Can you work these out from the model? Positions are in its coordinate system, mm. A direction names the side the tool comes from. Give positions to 0.01 mm unless a question says otherwise; leave off trailing zeros. Write each loop counter-clockwise with the first axis right and the second up, starting at its lowest first coordinate (ties: lowest second). Pieces come first, ordered by that corner, then holes. Notation, with made-up numbers: (20.5, -11.5) - (73.5, -11.5) arc R18 ccw to (73.5, -5.5) - close; hole circle Ø10 at (-23.5, -3.75). An arc over 180 degrees is marked (long way). Return JSON: item names as keys, results as strings. Group by question number.
from build123d import *

# Parameters (mm, degrees)
F1_R     = 7.5
F1_W     = 13
F1_H     = 13
F2_DEPTH = 5


with BuildPart() as f2:
    # F1 (on Right) → F2 (new body)
    with BuildSketch(Plane.YZ):
        Polygon((0, 15), (0, 0), (30, 0), (30, -5), (35, -5), (35, 0), (43.5, 0), (43.5, 2), (42.25, 2), (42.25, 5), (43.5, 5), (43.5, 6), (46.5, 6), (46.5, 5), (47.75, 5), (47.75, 2), (46.5, 2), (46.5, 0), (55, 0), (55, -5), (60, -5), (60, 0), (90, 0), (90, 15), (95, 15), (95, 20), (90, 20), (90, 28.5), (88, 28.5), (88, 27.25), (85, 27.25), (85, 28.5), (84, 28.5), (84, 31.5), (85, 31.5), (85, 32.75), (88, 32.75), (88, 31.5), (90, 31.5), (90, 40), (95, 40), (95, 45), (90, 45), (90, 60), (60, 60), (60, 65), (55, 65), (55, 60), (46.5, 60), (46.5, 58), (47.75, 58), (47.75, 55), (46.5, 55), (46.5, 54), (43.5, 54), (43.5, 55), (42.25, 55), (42.25, 58), (43.5, 58), (43.5, 60), (35, 60), (35, 65), (30, 65), (30, 60), (0, 60), (0, 45), (-5, 45), (-5, 40), (0, 40), (0, 31.5), (2, 31.5), (2, 32.75), (5, 32.75), (5, 31.5), (6, 31.5), (6, 28.5), (5, 28.5), (5, 27.25), (2, 27.25), (2, 28.5), (0, 28.5), (0, 20), (-5, 20), (-5, 15), align=None)
        with Locations((20, 22)):
            Circle(F1_R, mode=Mode.SUBTRACT)
        with Locations((55.75, 13)):
            Rectangle(F1_W, F1_H, mode=Mode.SUBTRACT)
        with BuildLine():
            Line((25, 50), (65, 50))
            ThreePointArc((65, 50), (70, 45), (65, 40))
            Line((65, 40), (25, 40))
            ThreePointArc((25, 40), (20, 45), (25, 50))
        make_face(mode=Mode.SUBTRACT)
    extrude(amount=F2_DEPTH)


solid = f2.part
1) Imagine slicing it at B-B, the plane y = 66. Write out the boundary of the cut face in (x, z), and give its area (3 significant figures).
2) Will these pins go through, and if not, where does the flat tip stop? pin 1 Ø2.5 at (x, y) = (3.5, 42.5) entering from +Z; pin 2 Ø1.5 at (x, y) = (2, 3) entering from -Z; pin 3 Ø2.5 at (x, z) = (3, 56) entering from -Y; pin 4 Ø5 at (y, z) = (17.5, 52) entering from -X.
3) On a 3-axis mill with a long thin cutter (end or side, diameter ignored), from which of +Z, -Z, +X, -X, +Y, -Y can I reach the whole of each face in a straight line? I mean faces 1 (the face through (2, 56, 19.5)), 2 (the face through (2, -2, 20)), 3 (the face through (2, 0, 53)). Say none if no direction works.
4) I need wall thicknesses on line 1 along Z through (x, y) = (1.5, 51); line 2 along Z through (x, y) = (1.55, 56); line 3 along Z through (x, y) = (3.1, 37). Which ranges of each line are inside material? Lowest first, please.
5) We'd pull the mould along Y, two halves only. Please class faces 4 (the face through (2, 57, -5)), 5 (the face through (2, 55, -2)), 6 (the face through (2, 43.5, 1)), 7 (the face through (2, 84, 30)): pulls with the +Y half, pulls with the -Y half, needs draft (parallel to the pull), parting line crosses it, or undercut.
6) Imagine slicing it at C-C, the plane x = 3.2. Count the separate pieces of the cut face and the enclosed holes in it, and give its area (3 significant figures).
7) Imagine slicing it at A-A, the plane z = 22. Write out the boundary of the cut face in (x, y), and give its area (3 significant figures).
Resolved:
{
 "1": {"outline": "(0, 0) - (5, 0) - (5, 40.1) - (0, 40.1) - close; (0, 49.9) - (5, 49.9) - (5, 60) - (0, 60) - close", "area": "251 mm^2"},
 "2": {"pin 1": "z = 60", "pin 2": "z = 0", "pin 3": "y = 0", "pin 4": "x = 0"},
 "3": {"face 1": "+X, -X", "face 2": "+X, -X, -Y", "face 3": "+Z, +X, -X, -Y"},
 "4": {"line 1": "0 to 6.5, 19.5 to 40, 50 to 60", "line 2": "-5 to 6.5, 19.5 to 40, 50 to 65", "line 3": "0 to 40, 50 to 60"},
 "5": {"face 4": "needs draft", "face 5": "undercut", "face 6": "undercut", "face 7": "pulls with the +Y half"},
 "6": {"separate pieces": "1", "enclosed holes": "3", "area": "4,670 mm^2"},
 "7": {"outline": "(0, 0) - (5, 0) - (5, 12.5) - (0, 12.5) - close; (0, 27.5) - (5, 27.5) - (5, 90) - (0, 90) - close", "area": "375 mm^2"}
}
